Can you work these out from the model? Positions are in its coordinate system, mm. Face numbers are marked on the shaded views. A direction names the side the tool comes from. Round coordinates to 2 decimals unless told otherwise and drop trailing zeros. Loops run counter-clockwise (first coordinate to the right, second up) from the corner with the lowest first, then second, coordinate; pieces in that order, holes last. Notation, with made-up numbers: (-21, 1.25) -> (-13, 1.25) arc R12 ccw to (-13, 8.25) -> close; hole circle Ø3 at (36.25, 71.25). An arc over 180 degrees is marked (long way). Write each question's results on one line, items separated by ' | '.
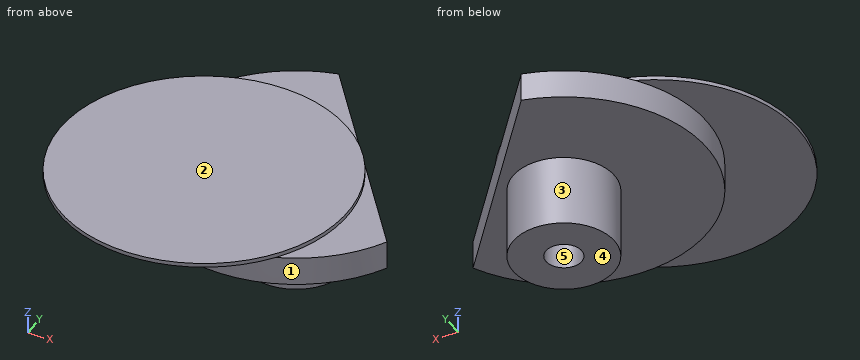
from build123d import *

# Parameters (mm, degrees)
F0_R     = 4.4958
F0_R_2   = 1.5875
F1_DEPTH = 6.35
F2_R     = 12.7
F3_DEPTH = 2.54
F5_DEPTH = 2.541
F6_R     = 12.7
F7_DEPTH = 0.3556


with BuildPart() as f1:
    # F0 (on Top) → F1 (new body)
    with BuildSketch(Plane.XY):
        Circle(F0_R)
        Circle(F0_R_2, mode=Mode.SUBTRACT)
    extrude(amount=F1_DEPTH)

    # F2 (on face) → F3 (join)
    with BuildSketch(Plane.XY.offset(6.35)):
        Circle(F2_R)
    extrude(amount=F3_DEPTH)

    # F4 (on face) → F5 (cut, through all)
    with BuildSketch(Plane(origin=(0, 0, 6.35), x_dir=(1, 0, 0), z_dir=(0, 0, -1))):
        Polygon((21.399127, -20.925693), (19.316025, 15.433881), (-10.036758, -20.925693), align=None)
    extrude(amount=-F5_DEPTH, mode=Mode.SUBTRACT)

    # F6 (on face) → F7 (join)
    with BuildSketch(Plane.XY.offset(8.89)):
        with Locations((-5.730732, -4.626373)):
            Circle(F6_R)
    extrude(amount=F7_DEPTH)


solid = f1.part
1. If we section it at A-A (z = 4): List the corners of the cut face in (x, y) for me (1 decimal).
Final values:
outline: circle Ø9 at (0, 0); hole circle Ø3.2 at (0, 0)
2. If we section it at B-B (y = -11.25): List the corners of the cut face in (x, z) for me, then the cut area to 3 significant figures.
Final values:
outline: (-16.57, 8.89) -> (-5.89, 8.89) -> (-5.89, 6.35) -> (5.89, 6.35) -> (5.89, 8.89) -> (5.11, 8.89) -> (5.11, 9.25) -> (-16.57, 9.25) -> close | area: 37.6 mm2
3. If we section it at C-C (x = 0): List the corners of the cut face in (y, z) for me, then the cut area to 3 significant figures.
Final values:
outline: (-15.96, 8.89) -> (-12.7, 8.89) -> (-12.7, 6.35) -> (-4.5, 6.35) -> (-4.5, 0) -> (-1.59, 0) -> (-1.59, 6.35) -> (1.59, 6.35) -> (1.59, 0) -> (4.5, 0) -> (4.5, 6.35) -> (8.49, 6.35) -> (8.49, 8.89) -> (6.71, 8.89) -> (6.71, 9.25) -> (-15.96, 9.25) -> close | area: 98.8 mm2
4. Will these pins go through, and if not, where does the flat tip stop? pin 1 (3 mm diameter, centred on x = -12, y = 9.5, fed in from +Z); pin 2 (1 mm diameter, centred on x = 0.5, y = 0.5, fed in from -Z).
Final values:
pin 1: through | pin 2: z = 6.35
5. If we section it at D-D (z = 7.25): List the corners of the cut face in (x, y) for me, then the cut area to 3 significant figures.
Final values:
outline: (-3.09, 12.32) arc R12.7 ccw (long way) to (11.39, -5.62) -> close | area: 385 mm2
6. On a 3-axis mill with a long thin cutter (end or side, diameter ignored), from which of +Z, -Z, +X, -X, +Y, -Y can I reach the whole of each face in a straight line? I mean the marked faces 1 and 2. Say none if no direction works.
Final values:
face 1: -Z | face 2: +Z, +X, -X, +Y, -Y
7. Please list where these lines run through material, in increasing order: line 1 (Y direction, x = 0, z = 2); line 2 (Z direction, x = -6.75, y = -4.25); line 3 (X direction, y = 1.25, z = 2.75). Write a range as from..to.
Final values:
line 1: -4.5..-1.59, 1.59..4.5 | line 2: 6.35..9.25 | line 3: -4.32..-0.98, 0.98..4.32
8. We'd pull the mould along Y, two halves only. Please class the marked faces 3, 4 and 5: pulls with the +Y half, pulls with the -Y half, needs draft (parallel to the pull), parting line crosses it, or undercut.
Final values:
face 3: parting line crosses it | face 4: needs draft | face 5: undercut
